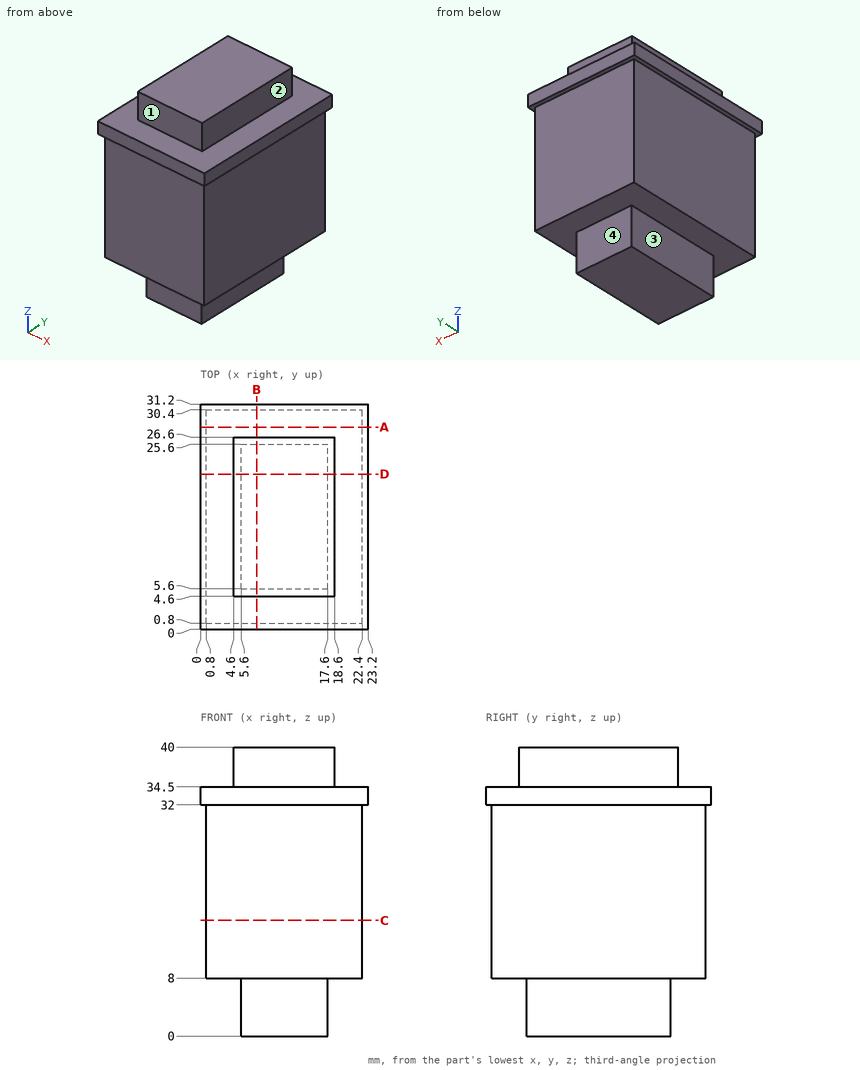
Here's the drawing with two shaded views (mm, measured from the low corner). I have some questions. A direction names the side the tool comes from. Coordinates: 2 decimals unless noted, no trailing zeros. Loops run counter-clockwise (first coordinate to the right, second up) from the corner with the lowest first, then second, coordinate; pieces in that order, holes last. Notation, with made-up numbers: (-21.75, 22.25) -> (-9.75, 22.25) arc R21 cw to (-9.75, 55.25) -> close; hole circle Ø6 at (31, 42). An arc over 180 degrees is marked (long way). Answer in a Markdown table with one row per item.
(1) Imagine slicing it at B-B (x = 7.75). List the corners of the cut face in (y, z) for me.
Results found:
| item | result |
|---|---|
| outline | (0, 32) -> (0.8, 32) -> (0.8, 8) -> (5.6, 8) -> (5.6, 0) -> (25.6, 0) -> (25.6, 8) -> (30.4, 8) -> (30.4, 32) -> (31.2, 32) -> (31.2, 34.5) -> (26.6, 34.5) -> (26.6, 40) -> (4.6, 40) -> (4.6, 34.5) -> (0, 34.5) -> close |
(2) Imagine slicing it at C-C (z = 16). List the corners of the cut face in (x, y) for me, plus the area to 3 significant figures.
Results found:
| item | result |
|---|---|
| outline | (0.8, 0.8) -> (22.4, 0.8) -> (22.4, 30.4) -> (0.8, 30.4) -> close |
| area | 639 mm^2 |
(3) Will these pins go through, and if not, where does the flat tip stop? pin 1 Ø3 at (x, z) = (12.5, 38) entering from +Y; pin 2 Ø6 at (y, z) = (16, 36) entering from -X; pin 3 Ø6.5 at (x, z) = (9.5, 5.5) entering from -Y; pin 4 Ø9 at (y, z) = (16.5, 4) entering from +X.
Results found:
| item | result |
|---|---|
| pin 1 | stops at y = 26.6 |
| pin 2 | stops at x = 0 |
| pin 3 | stops at y = 0.8 |
| pin 4 | stops at x = 22.4 |
(4) Imagine slicing it at D-D (y = 21.5). List the corners of the cut face in (x, z) for me.
Results found:
| item | result |
|---|---|
| outline | (0, 32) -> (0.8, 32) -> (0.8, 8) -> (5.6, 8) -> (5.6, 0) -> (17.6, 0) -> (17.6, 8) -> (22.4, 8) -> (22.4, 32) -> (23.2, 32) -> (23.2, 34.5) -> (18.6, 34.5) -> (18.6, 40) -> (4.6, 40) -> (4.6, 34.5) -> (0, 34.5) -> close |
(5) For the marked faces 1, 2, 3 and 4, which set-ups out of +Z, -Z, +X, -X, +Y, -Y let a thin tool reach every point of the face, with its end or its side?
Results found:
| item | result |
|---|---|
| face 1 | +Z, +X, -X, -Y |
| face 2 | +Z, +X, +Y, -Y |
| face 3 | -Z, -X, +Y, -Y |
| face 4 | -Z, +X, -X, +Y |
(6) Imagine slicing it at A-A (y = 28). List the corners of the cut face in (x, z) for me, plus the area to 3 significant figures.
Results found:
| item | result |
|---|---|
| outline | (0, 32) -> (0.8, 32) -> (0.8, 8) -> (22.4, 8) -> (22.4, 32) -> (23.2, 32) -> (23.2, 34.5) -> (0, 34.5) -> close |
| area | 576 mm^2 |
(7) If I drill on probe 1 along X at (y, z) = (4, 16.5); probe 2 along Z at (x, y) = (20.25, 13.5); probe 3 along Y at (x, z) = (9.25, 19), over which ranges is the centre line in solid material (lowest first)?
Results found:
| item | result |
|---|---|
| probe 1 | x = 0.8 to 22.4 |
| probe 2 | z = 8 to 34.5 |
| probe 3 | y = 0.8 to 30.4 |
